For this review, use the dimensioned drawing (mm, ordinates from the lowest corner) and the shaded views. A direction names the side the tool comes from. Coordinates: 2 decimals unless noted, no trailing zeros. Write each loop counter-clockwise with the first axis right and the second up, starting at its lowest first coordinate (ties: lowest second). Pieces come first, ordered by that corner, then holes. Notation, with made-up numbers: (3, 11.25) -> (10, 11.25) arc R8 ccw to (10, 16.25) -> close; hole circle Ø1 at (-33, 43.25). An arc over 180 degrees is marked (long way). Put each result on its own line as item: value. Start each with the question number.
Item 1: For the marked faces 1, 2 and 3, list the 3-axis set-ups (+Z, -Z, +X, -X, +Y, -Y) from which the entire face can be reached by the end or side of a thin tool; tool diameter is ignored.
Item 2: Consider section D-D on x = 17.2. Give the boundary of the cut face in (y, z), and give its area (3 significant figures).
Item 3: To check wall thickness, follow L1, parallel to X at y = 17.7, z = 6.25; L2, parallel to Y at x = 11.5, z = 3; L3, parallel to Z at x = 2, y = 17. State the ranges of each line that lie inside material, in increasing order.
Item 4: Insertion check: P1, Ø5, axis at x = 29, z = 8, coming from the +Y side; P2, Ø0.8, axis at y = 5, z = 7, coming from the -X side; P3, Ø1.4, axis at x = 1, z = 5.5, coming from the +Y side. Each pin has a flat end and moves straight along its axis. Give the tip position at first contact, or say it passes through.
Item 5: Consider section A-A on x = 29.8. Give the boundary of the cut face in (y, z), and give its area (3 significant figures).
Item 6: Consider section B-B on x = 2.8. Give the boundary of the cut face in (y, z).
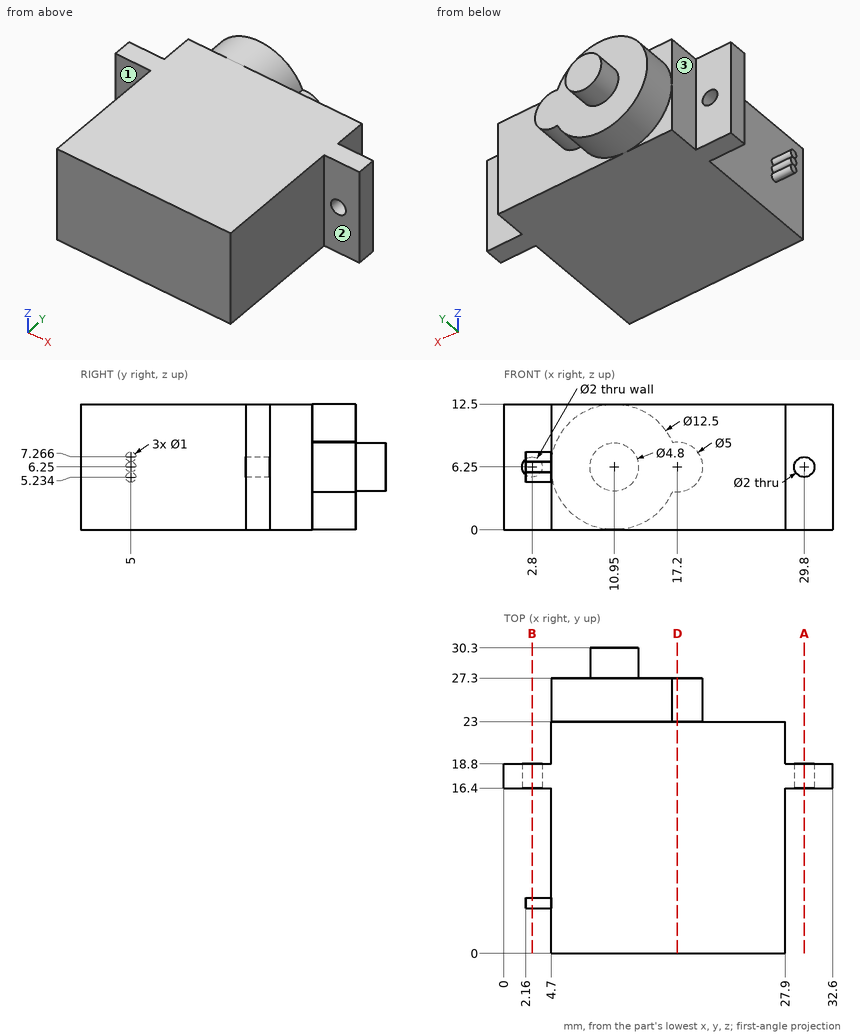
Return value:
1. face 1: +Z, -Z, -X
1. face 2: +Z, -Z, +X, -Y
1. face 3: +Z, -Z, -X, +Y
2. outline: (0, 0) -> (23, 0) -> (23, 3.75) -> (27.3, 3.75) -> (27.3, 8.75) -> (23, 8.75) -> (23, 12.5) -> (0, 12.5) -> close
2. area: 309 mm^2
3. L1: 0 to 1.8, 3.8 to 28.8, 30.8 to 32.6
3. L2: 0 to 27.3
3. L3: 0 to 5.65, 6.85 to 12.5
4. P1: y = 23
4. P2: x = 2.16
4. P3: y = 18.8
5. outline: (16.4, 0) -> (18.8, 0) -> (18.8, 5.25) -> (16.4, 5.25) -> close; (16.4, 7.25) -> (18.8, 7.25) -> (18.8, 12.5) -> (16.4, 12.5) -> close
5. area: 25.2 mm^2
6. outline: circle Ø1 at (5, 5.23); circle Ø1 at (5, 6.25); circle Ø1 at (5, 7.27); (16.4, 0) -> (18.8, 0) -> (18.8, 5.25) -> (16.4, 5.25) -> close; (16.4, 7.25) -> (18.8, 7.25) -> (18.8, 12.5) -> (16.4, 12.5) -> close
